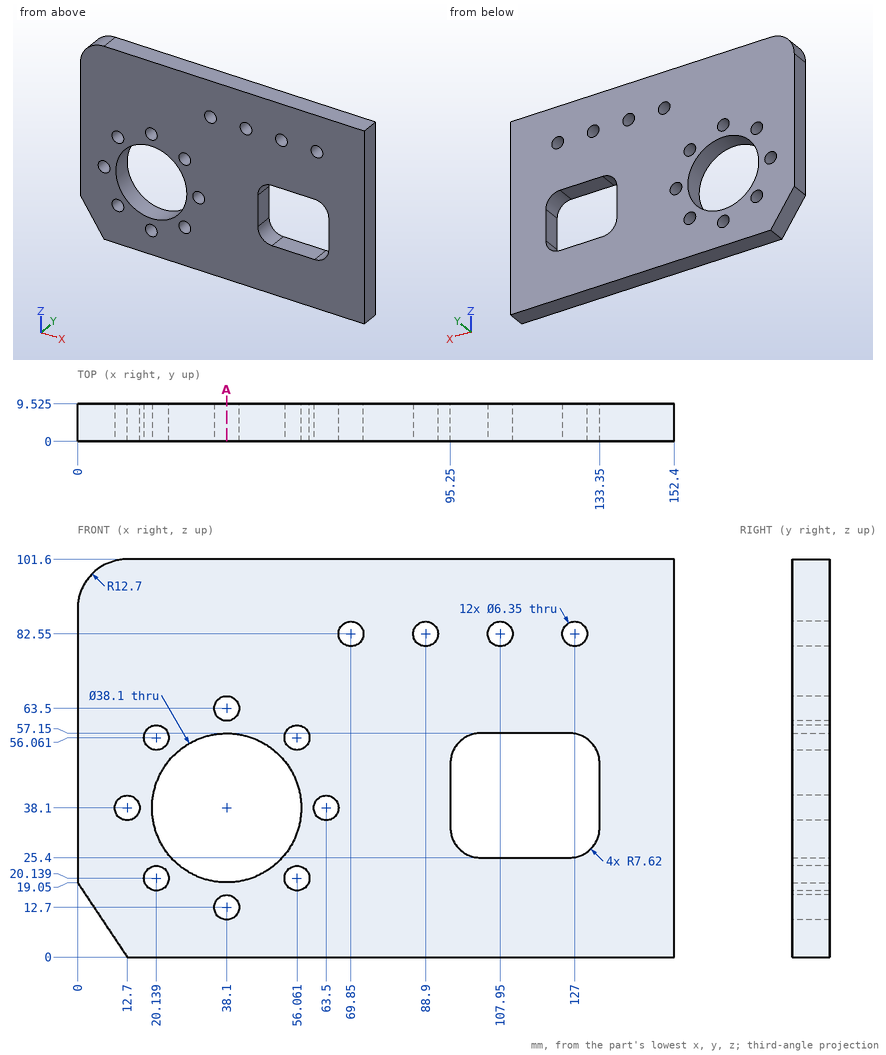
Source: three-view drawing plus pictorial views. Frame: mm from the lowest corner of the part. Round coordinates to 2 decimals unless told otherwise and drop trailing zeros. Put each result on its own line as item: value. Start each with the question number.
(1) Section query A-A (x = 38.1). State how many separate pieces and enclosed holes the cut face has, then the cut area to 3 significant figures.
(2) Contact query for flat-ended pins moving along their axis: pin 1 Ø5 at (x, z) = (56.06, 56.06) entering from +Y; pin 2 Ø8.5 at (x, z) = (69.85, 82.55) entering from +Y (1 decimal). Output: stop coordinate, or through.
(3) Material intervals for line 1 along X through (y, z) = (2.5, 82.55) (1 decimal); line 2 along Z through (x, y) = (89, 1.25); line 3 along X through (y, z) = (2.5, 54) (1 decimal), sorted ascending. Write a range as [from, to].
Findings below:
1. separate pieces: 4
1. enclosed holes: 0
1. area: 484 mm2
2. pin 1: passes through
2. pin 2: stops at y = 9.5
3. line 1: x = [0, 66.7], [73, 85.7], [92.1, 104.8], [111.1, 123.8], [130.2, 152.4]
3. line 2: z = [0, 79.38], [85.72, 101.6]
3. line 3: x = [0, 17.7], [22.6, 27.6], [48.6, 53.6], [58.5, 96.7], [131.9, 152.4]
